```python
from build123d import *

# Parameters (mm, degrees)
F0_R      = 38.1
F1_DEPTH  = 40
F2_R      = 12.7
F3_DEPTH  = 35
F4_SIZE   = 5
F11_R     = 3.4
F12_DEPTH = 50
F15_SIZE  = 2
F16_R     = 3.4
F17_DEPTH = 50
F18_R     = 3.4
F19_DEPTH = 50


with BuildPart() as f1:
    # F0 (on Top) → F1 (new body)
    with BuildSketch(Plane.XY):
        Circle(F0_R)
    extrude(amount=F1_DEPTH)

    # F2 (on face) → F3 (cut)
    with BuildSketch(Plane.XY.offset(40)):
        Circle(F2_R)
    extrude(amount=-F3_DEPTH, mode=Mode.SUBTRACT)

    # F4
    f4_edges = [f1.edges().sort_by_distance(p)[0] for p in [
        (-38.1, 0, 40),
    ]]
    chamfer(f4_edges, length=F4_SIZE)

    # F11 (on face) → F12 (cut)
    with BuildSketch(Plane(origin=(46.512412, -46.512412, -23.94141), x_dir=(0.747321, 0.590792, 0.304099), z_dir=(0.664463, -0.664463, -0.34202))):
        with Locations((6.472312, 18.923773)):
            Circle(F11_R)
    extrude(amount=-F12_DEPTH, mode=Mode.SUBTRACT)

    # F15
    f15_edges = [f1.edges().sort_by_distance(p)[0] for p in [
        (-38.1, 0, 0),
    ]]
    chamfer(f15_edges, length=F15_SIZE)

    # F16 (on face) → F17 (cut)
    with BuildSketch(Plane(origin=(46.512412, 46.512412, -23.94141), x_dir=(-0.747321, 0.590792, -0.304099), z_dir=(0.664463, 0.664463, -0.34202))):
        with Locations((-6.472312, 18.923773)):
            Circle(F16_R)
    extrude(amount=-F17_DEPTH, mode=Mode.SUBTRACT)

    # F18 (on face) → F19 (cut)
    with BuildSketch(Plane(origin=(-60.04, 0, -13.310548), x_dir=(0, -1, 0), z_dir=(-0.976296, 0, -0.21644))):
        with Locations((0, 15)):
            Circle(F18_R)
    extrude(amount=-F19_DEPTH, mode=Mode.SUBTRACT)


solid = f1.part
```
For this review, take the finished solid that the model builds, in its own axes (mm). A direction names the side the tool comes from. Give positions to 0.01 mm unless a question says otherwise; leave off trailing zeros. Order: outer loops, then holes, each group sorted by start corner. A loop starts at its lowest first (then second) coordinate and runs counter-clockwise, first axis right, second up.
1) Take a section at C-C (z = 21). Give the boundary of the cut face in (x, y).
2) The part is to be moulded in two halves that separate along Z. For faces 1 (the face through (21.84, 22.56, 6.28)), 2 (the face through (-2.75, -12.4, 22.74)), 3 (the face through (0, 0, 5)), say which applies: released by +Z, released by -Z, zero draft, split by the parting line, or undercut.
3) Take a section at A-A (x = 0). Give the boundary of the cut face in (y, z).
4) Take a section at B-B (y = 0). Give the boundary of the cut face in (x, z), then the cut area to 3 significant figures.
5) Insertion check: pin 1 (20.5 mm diameter, centred on x = 0, y = 0, fed in from +Z); pin 2 (5 mm diameter, centred on x = -22, z = 17.5, fed in from +Y); pin 3 (6 mm diameter, centred on x = -19, z = 21.5, fed in from -Y). Each pin has a flat end and moves straight along its axis. Give the tip position at first contact, or say it passes through.
6) For faces 4 (the face through (36.34, 11.44, 18.27)), 5 (the face through (18.091, -18.176, 11.981)), list the 3-axis set-ups (+Z, -Z, +X, -X, +Y, -Y) from which the entire face can be reached by the end or side of a thin tool; tool diameter is ignored.
7) Wall thickness on line 1 (Y direction, x = 0, z = 17); line 2 (X direction, y = -7.5, z = 35.5); line 3 (Z direction, x = 11, y = 5): over which ranges is each line inside the solid? List them lowest first.
Derived:
1. outline: circle Ø76.2 at (0, 0); hole circle Ø25.4 at (0, 0)
2. face 1: undercut
2. face 2: zero draft
2. face 3: released by +Z
3. outline: (-38.1, 2) - (-36.1, 0) - (36.1, 0) - (38.1, 2) - (38.1, 35) - (33.1, 40) - (12.7, 40) - (12.7, 5) - (-12.7, 5) - (-12.7, 40) - (-33.1, 40) - (-38.1, 35) - close
4. outline: (-38.1, 2) - (-36.1, 0) - (36.1, 0) - (38.1, 2) - (38.1, 35) - (33.1, 40) - (12.7, 40) - (12.7, 5) - (-12.7, 5) - (-12.7, 40) - (-33.1, 40) - (-38.1, 35) - (-38.1, 10.4) - (-15.21, 15.48) - (-13.74, 8.84) - (-38.1, 3.44) - close
4. area: 1,970 mm2
5. pin 1: stops at z = 5
5. pin 2: stops at y = 32.73
5. pin 3: stops at y = -34.58
6. face 4: +Z, -Z
6. face 5: none
7. line 1: y = -38.1 to -12.7, 12.7 to 38.1
7. line 2: x = -36.84 to -10.25, 10.25 to 36.84
7. line 3: z = 0 to 5
